Can you work these out from the model? Positions are in its coordinate system, mm. A direction names the side the tool comes from. Give positions to 0.01 mm unless a question says otherwise; leave off trailing zeros. Order: outer loops, then holes, each group sorted by start corner. A loop starts at its lowest first (then second) coordinate and runs counter-clockwise, first axis right, second up. Notation, with made-up numbers: M 71.25,-7 L 110.25,-7 A28 cw 110.25,23 Z; hole C 43.5,-8.5 d10. An arc over 180 degrees is marked long. Use one line per item in the form item = value. Start each with the question number.
1. I want a section at A-A, the plane x = 0. List the corners of the cut face in (y, z) for me.
2. I need wall thicknesses on L1, parallel to Z at x = 12.5, y = 18; L2, parallel to Y at x = -6.5, z = 6.75; L3, parallel to X at y = -9, z = 10.5. Which ranges of each line are inside material? Lowest first, please.
3. I want a section at C-C, the plane z = 1.75. List the corners of the cut face in (x, y) for me, and give its area (3 significant figures).
4. I want a section at D-D, the plane z = 11.75. List the corners of the cut face in (x, y) for me.
5. Will these pins go through, and if not, where does the flat tip stop? P1, Ø2, axis at y = -12.5, z = 7, coming from the +X side; P2, Ø10, axis at y = -19.5, z = 7.5, coming from the +X side; P3, Ø10, axis at x = 17.5, y = -28, coming from the +Z side; P4, Ø4, axis at y = 2, z = 13.5, coming from the -X side.
6. For faces 1 (the face through (6.691, -12.864, 9.93)), 2 (the face through (0, 0, 20)), which set-ups out of +Z, -Z, +X, -X, +Y, -Y let a thin tool reach every point of the face, with its end or its side?
```python
from build123d import *

# Parameters (mm, degrees)
F0_R     = 14.5
F1_DEPTH = 20
F0_W     = 105
F0_H     = 105
F2_DEPTH = 5
F3_R     = 15
F4_SIZE  = 5


with BuildPart() as f1:
    # F0 (on Top) → F1 (new body)
    with BuildSketch(Plane.XY):
        Circle(F0_R)
    extrude(amount=F1_DEPTH)

    # F0 (on Top) → F2 (join)
    with BuildSketch(Plane.XY):
        Rectangle(F0_W, F0_H)
        Circle(F0_R, mode=Mode.SUBTRACT)
    extrude(amount=F2_DEPTH)

    # F3
    f3_edges = [f1.edges().sort_by_distance(p)[0] for p in [
        (52.5, -52.5, 2.5),
        (-52.5, -52.5, 2.5),
        (-52.5, 52.5, 2.5),
        (52.5, 52.5, 2.5),
    ]]
    fillet(f3_edges, radius=F3_R)

    # F4
    f4_edges = [f1.edges().sort_by_distance(p)[0] for p in [
        (-14.5, 0, 20),
    ]]
    chamfer(f4_edges, length=F4_SIZE)


solid = f1.part
```
Check result:
q1.outline = M -52.5,0 L 52.5,0 L 52.5,5 L 14.5,5 L 14.5,15 L 9.5,20 L -9.5,20 L -14.5,15 L -14.5,5 L -52.5,5 Z
q2.L1 = 0 to 5
q2.L2 = -12.96 to 12.96
q2.L3 = -11.37 to 11.37
q3.outline = M -52.5,-37.5 A15 ccw -37.5,-52.5 L 37.5,-52.5 A15 ccw 52.5,-37.5 L 52.5,37.5 A15 ccw 37.5,52.5 L -37.5,52.5 A15 ccw -52.5,37.5 Z
q3.area = 10,800 mm2
q4.outline = C 0,0 d29
q5.P1 = 8.83
q5.P2 = 52.5
q5.P3 = 5
q5.P4 = -14.5
q6.face_1 = +Z
q6.face_2 = +Z, +X, -X, +Y, -Y
